Autodesk Inventor part; units mm, degrees
ref_plane "YZ Plane" through (0, 0, 0) normal (1, 0, 0) x (0, 1, 0)
ref_plane "XZ Plane" through (0, 0, 0) normal (0, 1, 0) x (-1, 0, 0)
ref_plane "XY Plane" through (0, 0, 0) normal (0, 0, 1) x (1, 0, 0)
sketch "Sketch1" plane through (0, 0, 0) normal (0, 1, 0) x (-1, 0, 0)
  line L0 (16.5, -23.5) -> (-16.5, -23.5)
  line L1 (-16.5, -23.5) -> (-16.5, 23.5)
  line L2 (-16.5, 23.5) -> (16.5, 23.5)
  line L3 (16.5, 23.5) -> (16.5, -23.5)
  point P0 (0, 0)
  point P1 (16.5, 0)
  point P2 (0, -23.5)
  dimension "d0" = 33
  dimension "d1" = 47
extrude "Extrusion1" add sketch "Sketch1" along normal mid plane 2
sketch "Sketch2" plane through (0, 1, 0) normal (0, 1, 0) x (1, 0, 0)
  circle A0 centre (0, 0) radius 9
  line L0 (-8, -4.1231) -> (-8, 4.1231)
  line L1 (8, 4.1231) -> (8, -4.1231)
  line L2 (0, 32.9) -> (0, -32.9)
  dimension "d4" = 18
  dimension "d5" = 16
extrude "Extrusion2" cut sketch "Sketch2" against normal through all contours L1 A0 L2 | L2 A0 L0
sketch "Sketch3" plane through (0, 1, 0) normal (0, 1, 0) x (1, 0, 0)
  line L0 (-3.5, -8.2916) -> (-3.5, -14.5)
  arc A0 (-3.5, -14.5) -> (3.5, -14.5) centre (0, -14.5) ccw
  line L1 (3.5, -14.5) -> (3.5, -8.2916)
  line L2 (16.5, -3.5) -> (13.5, -3.5)
  arc A1 (13.5, 3.5) -> (13.5, -3.5) centre (13.5, 0) ccw
  line L3 (13.5, 3.5) -> (16.5, 3.5)
  line L4 (-16.5, 3.5) -> (-13.5, 3.5)
  arc A2 (-13.5, -3.5) -> (-13.5, 3.5) centre (-13.5, 0) ccw
  line L5 (-13.5, -3.5) -> (-16.5, -3.5)
  line L6 (8, 4.1231) -> (8, -4.1231)
  arc A3 (-8, -4.1231) -> (8, -4.1231) centre (0, 0) ccw
  line L7 (-8, -4.1231) -> (-8, 4.1231)
  arc A4 (8, 4.1231) -> (-8, 4.1231) centre (0, 0) ccw
  line L8 (16.5, 23.5) -> (16.5, -23.5)
  line L9 (-16.5, 23.5) -> (16.5, 23.5)
  line L10 (-16.5, -23.5) -> (-16.5, 23.5)
  line L11 (16.5, -23.5) -> (-16.5, -23.5)
  line L12 (-23.1, 0) -> (23.1, 0)
  line L13 (0, 32.9) -> (0, -32.9)
  dimension "d8" = 20
  dimension "d9" = 7
  dimension "d10" = 7
  dimension "d11" = 27
extrude "Extrusion3" cut sketch "Sketch3" against normal through all contours A3 L13 A0 L0 | A3 L1 A0 L13 | L12 L10 L4 A2 | A2 L5 L10 L12 | L12 L8 L2 A1 | A1 L3 L8 L12
fillet "Fillet1" radius 2 4 edges at (-16.5, 0, 23.5) (16.5, 0, 23.5) (16.5, 0, -23.5) (-16.5, 0, -23.5)
properties part number "Quick Release Rubber Pad" material "Rubber"
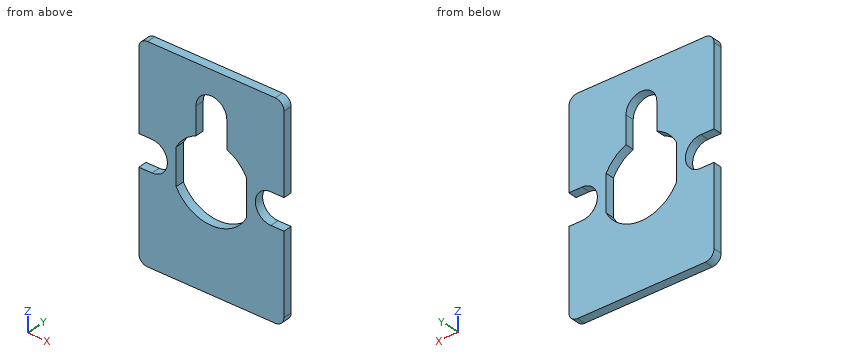
Here's how the part is built. I have some questions about the finished solid (model axes, mm). Coordinates: 2 decimals unless noted, no trailing zeros. Order: outer loops, then holes, each group sorted by start corner. A loop starts at its lowest first (then second) coordinate and runs counter-clockwise, first axis right, second up. Notation, with made-up numbers: (-12, -21) - (45, -21) arc R18 ccw to (45, 13) - close; hole circle Ø8 at (-28, -1.75). An arc over 180 degrees is marked (long way). Use CSV: the item, a comma, the result in double quotes. Start each with the question number.
1. I'm going to push flat-ended pins straight in: pin 1 (1 mm diameter, centred on x = 15, y = 0, fed in from -Z); pin 2 (0.6 mm diameter, centred on y = 0, z = 2, fed in from +X); pin 3 (1 mm diameter, centred on y = 0, z = 1, fed in from -X). Where does each tip first touch, or does it pass through?
2. Suppose I cut it at B-B on x = 0. List the corners of the cut face in (y, z) for me.
3. Suppose I cut it at C-C on y = -0.55. List the corners of the cut face in (x, z) for me, then the cut area to 3 significant figures.
4. Suppose I cut it at A-A on z = 14. List the corners of the cut face in (x, y) for me, then the cut area to 3 significant figures.
5. Please list where these lines run through material, in increasing order: line 1 (Z direction, x = 11, y = 0.25); line 2 (Z direction, x = 2, y = -0.8); line 3 (X direction, y = -0.85, z = 17.5). Write a range as from..to.
Output:
1,pin 1,"stops at z = -23.5"
1,pin 2,"stops at x = 10.86"
1,pin 3,"stops at x = -10.34"
2,outline,"(-1, -23.5) - (1, -23.5) - (1, -9) - (-1, -9) - close; (-1, 18) - (1, 18) - (1, 23.5) - (-1, 23.5) - close"
3,outline,"(-16.5, -21.5) arc R2 ccw to (-14.5, -23.5) - (14.5, -23.5) arc R2 ccw to (16.5, -21.5) - (16.5, -3.5) - (13.5, -3.5) arc R3.5 cw to (13.5, 3.5) - (16.5, 3.5) - (16.5, 21.5) arc R2 ccw to (14.5, 23.5) - (-14.5, 23.5) arc R2 ccw to (-16.5, 21.5) - (-16.5, 3.5) - (-13.5, 3.5) arc R3.5 cw to (-13.5, -3.5) - (-16.5, -3.5) - close; hole (-8, -4.12) arc R9 ccw to (8, -4.12) - (8, 4.12) arc R9 ccw to (3.5, 8.29) - (3.5, 14.5) arc R3.5 ccw to (-3.5, 14.5) - (-3.5, 8.29) arc R9 ccw to (-8, 4.12) - close"
3,area,"1,160 mm2"
4,outline,"(-16.5, -1) - (-3.5, -1) - (-3.5, 1) - (-16.5, 1) - close; (3.5, -1) - (16.5, -1) - (16.5, 1) - (3.5, 1) - close"
4,area,"52.0 mm2"
5,line 1,"z = -23.5..-2.45, 2.45..23.5"
5,line 2,"z = -23.5..-8.77, 17.37..23.5"
5,line 3,"x = -16.5..-1.8, 1.8..16.5"
